Geometry check sheet. Reference: drawing and pictorial views, mm from the part's lowest x, y, z. A direction names the side the tool comes from. Round coordinates to 2 decimals unless told otherwise and drop trailing zeros. Write each loop counter-clockwise with the first axis right and the second up, starting at its lowest first coordinate (ties: lowest second). Pieces come first, ordered by that corner, then holes.
Item 1: Material ranges on line 1 along Y through (x, z) = (4.75, 2.3); line 2 along X through (y, z) = (1.25, 1.45); line 3 along Y through (x, z) = (3.65, 1.7), recorded low to high.
Item 2: Section check D-D, the plane x = 6.25. Record the cut outline in (y, z), plus the area to 3 significant figures.
Item 3: Set-up check for the marked faces 1, 2, 3, 4 and 5: record each of +Z, -Z, +X, -X, +Y, -Y from which the full face is reachable in a straight line by a thin tool's end or side.
Item 4: Section check A-A, the plane y = 11.65. Record the cut outline in (x, z).
Item 5: Section check B-B, the plane x = 3.65. Record the cut outline in (y, z).
Item 6: Depth check by flat-ended pin: pin 1 (0.6 mm diameter, centred on x = 2.5, y = 14, fed in from +Z); pin 2 (1.5 mm diameter, centred on x = 4, y = 10, fed in from +Z); pin 3 (1.6 mm diameter, centred on x = 3, y = 14.5, fed in from -Z). Enter the tip coordinate at first touch or a pass-through.
Item 7: Section check C-C, the plane z = 1.45. Record the cut outline in (x, y).
Item 8: Release check for a two-part mould opening along Z. For the marked faces 6, 7, 8 and 9 record: pulls with the +Z half, pulls with the -Z half, needs draft (parallel to the pull), parting line crosses it, or undercut.
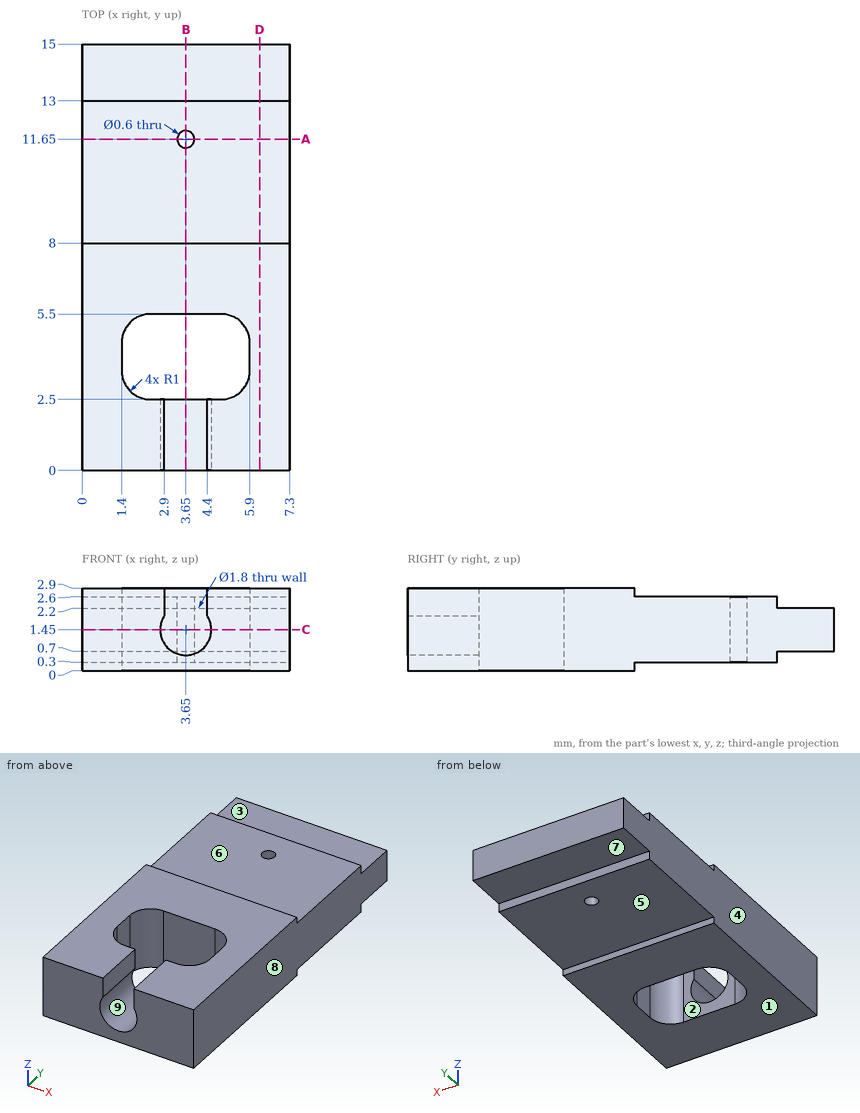
Values found:
1. line 1: y = 0 to 2.5, 5.5 to 13
1. line 2: x = 0 to 2.75, 4.55 to 7.3
1. line 3: y = 5.5 to 11.35, 11.95 to 15
2. outline: (0, 0) - (8, 0) - (8, 0.3) - (13, 0.3) - (13, 0.7) - (15, 0.7) - (15, 2.2) - (13, 2.2) - (13, 2.6) - (8, 2.6) - (8, 2.9) - (0, 2.9) - close
2. area: 37.7 mm2
3. face 1: -Z, +X, -X, +Y, -Y
3. face 2: +Z, -Z
3. face 3: +Z, +X, -X, +Y
3. face 4: +Z, -Z, -X, +Y, -Y
3. face 5: -Z, +X, -X, +Y
4. outline: (0, 0.3) - (3.35, 0.3) - (3.35, 2.6) - (0, 2.6) - close; (3.95, 0.3) - (7.3, 0.3) - (7.3, 2.6) - (3.95, 2.6) - close
5. outline: (0, 0) - (2.5, 0) - (2.5, 0.55) - (0, 0.55) - close; (5.5, 0) - (8, 0) - (8, 0.3) - (11.35, 0.3) - (11.35, 2.6) - (8, 2.6) - (8, 2.9) - (5.5, 2.9) - close; (11.95, 0.3) - (13, 0.3) - (13, 0.7) - (15, 0.7) - (15, 2.2) - (13, 2.2) - (13, 2.6) - (11.95, 2.6) - close
6. pin 1: stops at z = 2.2
6. pin 2: stops at z = 2.6
6. pin 3: stops at z = 0.7
7. outline: (0, 0) - (2.75, 0) - (2.75, 2.5) - (2.4, 2.5) arc R1 cw to (1.4, 3.5) - (1.4, 4.5) arc R1 cw to (2.4, 5.5) - (4.9, 5.5) arc R1 cw to (5.9, 4.5) - (5.9, 3.5) arc R1 cw to (4.9, 2.5) - (4.55, 2.5) - (4.55, 0) - (7.3, 0) - (7.3, 15) - (0, 15) - close; hole circle Ø0.6 at (3.65, 11.65)
8. face 6: pulls with the +Z half
8. face 7: pulls with the -Z half
8. face 8: needs draft
8. face 9: undercut
